Autodesk Inventor part; units mm, degrees
ref_plane "YZ Plane" through (0, 0, 0) normal (1, 0, 0) x (0, 1, 0)
ref_plane "XZ Plane" through (0, 0, 0) normal (0, 1, 0) x (-1, 0, 0)
ref_plane "XY Plane" through (0, 0, 0) normal (0, 0, 1) x (1, 0, 0)
sketch "Sketch1" plane through (0, 0, 0) normal (0, 0, 1) x (1, 0, 0)
  line L0 (0, 0) -> (25.4, 0)
  line L1 (25.4, 0) -> (25.4, 25.4)
  line L2 (25.4, 25.4) -> (0, 25.4)
  line L3 (0, 25.4) -> (0, 0)
  line L4 (3.175, 22.225) -> (22.225, 22.225)
  line L5 (22.225, 22.225) -> (22.225, 3.175)
  line L6 (22.225, 3.175) -> (3.175, 3.175)
  line L7 (3.175, 3.175) -> (3.175, 22.225)
  dimension "d0" = 25.4
  dimension "d1" = 25.4
  dimension "d2" = 3.175
extrude "Extrusion1" add sketch "Sketch1" along normal blind 584.2
sketch "Sketch2" plane through (25.4, 0, 0) normal (1, 0, 0) x (0, 0, -1)
  line L0 (0, 3.175) -> (0, 22.225) construction
  line L1 (0, 12.7) -> (-12.7, 12.7) construction
  line L2 (-12.7, 12.7) -> (-38.1, 12.7) construction
  line L3 (-584.2, 22.225) -> (-584.2, 3.175) construction
  line L4 (-584.2, 12.7) -> (-571.5, 12.7) construction
  line L5 (-571.5, 12.7) -> (-546.1, 12.7) construction
  circle A0 centre (-571.5, 12.7) radius 2.5797
  circle A1 centre (-546.1, 12.7) radius 2.5797
  circle A2 centre (-38.1, 12.7) radius 2.5797
  circle A3 centre (-12.7, 12.7) radius 2.5797
  point P0 (0, 0)
  dimension "d5" = 12.7
  dimension "d6" = 25.4
  dimension "d7" = 12.7
  dimension "d8" = 25.4
  dimension "d9" = 5.1594
  dimension "d18" = 5.1594
  dimension "d19" = 5.1594
  dimension "d20" = 5.1594
extrude "Extrusion2" cut sketch "Sketch2" against normal blind 584.2
sketch "Sketch3" plane through (25.4, 0, 0) normal (1, 0, 0) x (0, 0, -1)
  line L0 (-584.2, 22.225) -> (-584.2, 3.175) construction
  line L1 (-584.2, 12.7) -> (-393.7, 12.7) construction
  circle A0 centre (-393.7, 12.7) radius 2.5797
  line L2 (-393.7, 12.7) -> (-419.1, 12.7) construction
  line L3 (-419.1, 12.7) -> (-368.3, 12.7) construction
  circle A1 centre (-419.1, 12.7) radius 2.5797
  circle A2 centre (-368.3, 12.7) radius 2.5797
  line L4 (0, 25.4) -> (-584.2, 25.4) construction
  line L5 (-292.1, 25.4) -> (-292.1, 0) construction
  circle A3 centre (-190.5, 12.7) radius 2.5797
  circle A4 centre (-165.1, 12.7) radius 2.5797
  circle A5 centre (-215.9, 12.7) radius 2.5797
  point P0 (0, 0)
  dimension "d12" = 190.5
  dimension "d13" = 5.1594
  dimension "d14" = 25.4
  dimension "d15" = 50.8
extrude "Extrusion3" cut sketch "Sketch3" against normal blind 584.2
properties part number "1x1 23in"
The listing builds one solid part. Answer for the finished solid, in the listing's coordinates (mm). A direction names the side the tool comes from. Round coordinates to 2 decimals unless told otherwise and drop trailing zeros. Loops run counter-clockwise (first coordinate to the right, second up) from the corner with the lowest first, then second, coordinate; pieces in that order, holes last.
1) A cutting plane is placed at B-B on z = 457. Determine the outline of the cut face in (x, y) (3 decimals).
Outcome:
outline: (0, 0) - (25.4, 0) - (25.4, 25.4) - (0, 25.4) - close; hole (3.175, 3.175) - (22.225, 3.175) - (22.225, 22.225) - (3.175, 22.225) - close
2) A cutting plane is placed at A-A on x = 13.5. Determine the outline of the cut face in (y, z) (3 decimals).
Outcome:
outline: (0, 0) - (3.175, 0) - (3.175, 584.2) - (0, 584.2) - close; (22.225, 0) - (25.4, 0) - (25.4, 584.2) - (22.225, 584.2) - close
3) For faces 1 (the face through (13, 3.175, 288)), 2 (the face through (13, 0, 288)), determine the directions among +Z, -Z, +X, -X, +Y, -Y from which every point of the face is accessible in a straight line to the end or side of a thin tool.
Outcome:
face 1: +Z, -Z
face 2: +Z, -Z, +X, -X, -Y
4) For a pull along Y with two mould halves and no side action, classify faces 3 (the face through (13, 25.4, 288)), 4 (the face through (25.4, 13, 288)), 5 (the face through (3.175, 13, 288)) as released by +Y, released by -Y, zero draft, split by the parting line, or undercut.
Outcome:
face 3: released by +Y
face 4: zero draft
face 5: undercut
5) Given P1, Ø3, axis at y = 12.7, z = 546.1, coming from the +X side, flat-ended and moving along its own axis, determine where the tip first touches the part or whether it passes through.
Outcome:
P1: passes through
6) Consider line 1 (Y direction, x = 8.75, z = 425.5) (3 decimals); line 2 (Y direction, x = 2.3, z = 215.9). Determine where each line is inside the solid, lowest interval first.
Outcome:
line 1: y = 0 to 3.175, 22.225 to 25.4
line 2: y = 0 to 10.12, 15.28 to 25.4
